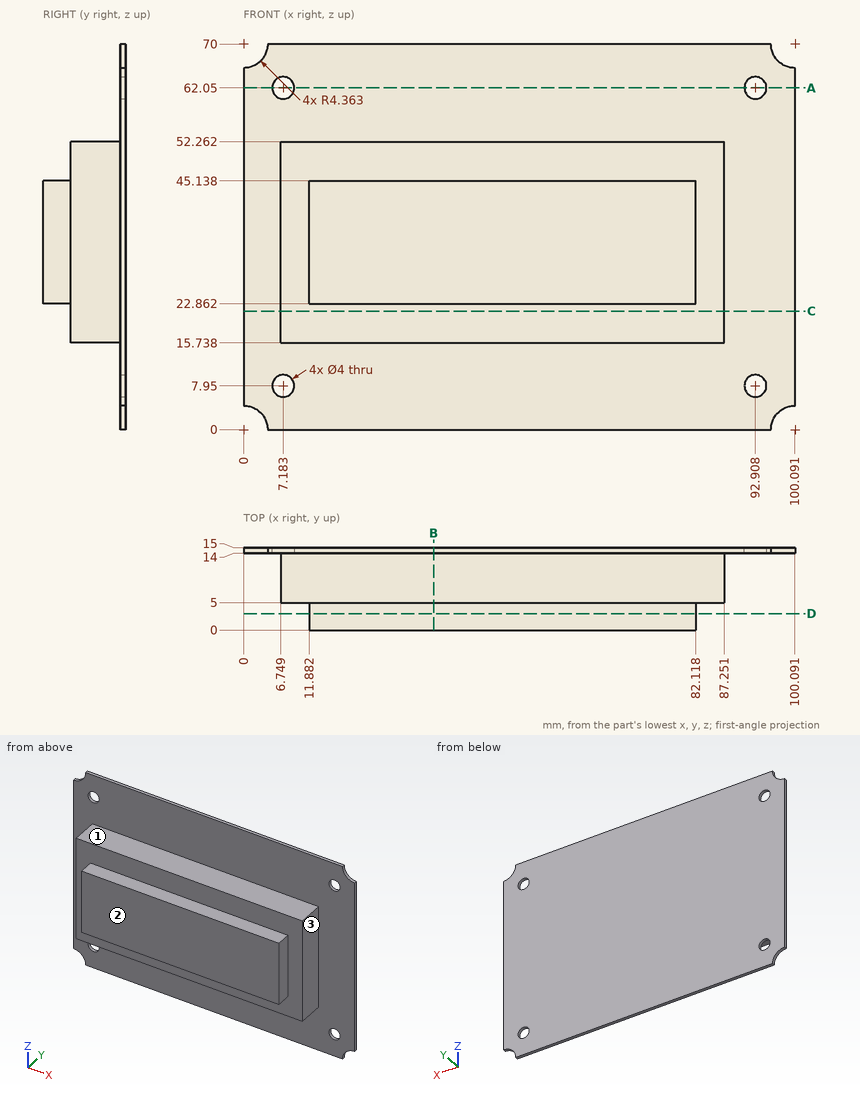
Source: three-view drawing plus pictorial views. Frame: mm from the lowest corner of the part. A direction names the side the tool comes from. Coordinates: 2 decimals unless noted, no trailing zeros. Order: outer loops, then holes, each group sorted by start corner. A loop starts at its lowest first (then second) coordinate and runs counter-clockwise, first axis right, second up.
1) Section A-A (z = 62.05). Return loops of the section in (x, y).
Result sheet:
outline: (0, 14) - (5.18, 14) - (5.18, 15) - (0, 15) - close; (9.18, 14) - (90.91, 14) - (90.91, 15) - (9.18, 15) - close; (94.91, 14) - (100.09, 14) - (100.09, 15) - (94.91, 15) - close
2) Ray query, probe 1 along Z at (x, y) = (84, 12.25); probe 2 along X at (y, z) = (13, 27.5); probe 3 along Y at (x, z) = (75.5, 4.5). Return the intervals inside material, ascending.
Result sheet:
probe 1: z = 15.74 to 52.26
probe 2: x = 6.75 to 87.25
probe 3: y = 14 to 15
3) Section C-C (z = 21.5). Return loops of the section in (x, y).
Result sheet:
outline: (0, 14) - (6.75, 14) - (6.75, 5) - (87.25, 5) - (87.25, 14) - (100.09, 14) - (100.09, 15) - (0, 15) - close
4) Section D-D (y = 3). Return loops of the section in (x, z), then the cut area to 3 significant figures.
Result sheet:
outline: (11.88, 22.86) - (82.12, 22.86) - (82.12, 45.14) - (11.88, 45.14) - close
area: 1,560 mm2
5) Section B-B (x = 34.5). Return loops of the section in (y, z).
Result sheet:
outline: (0, 22.86) - (5, 22.86) - (5, 15.74) - (14, 15.74) - (14, 0) - (15, 0) - (15, 70) - (14, 70) - (14, 52.26) - (5, 52.26) - (5, 45.14) - (0, 45.14) - close
6) First-contact query: P1, Ø4.5, axis at x = 45, y = 9.5, coming from the -Z side; P2, Ø1.5, axis at x = 48.5, y = 2, coming from the +Z side; P3, Ø4, axis at y = 1.5, z = 39.5, coming from the +X side. Flat tips, straight axial feed; report the tip coordinate or a pass-through.
Result sheet:
P1: stops at z = 15.74
P2: stops at z = 45.14
P3: stops at x = 82.12
7) Set-up query: the marked faces 1, 2 and 3. Return all of +Z, -Z, +X, -X, +Y, -Y with unobstructed straight access to the full face (end or side cutting, diameter ignored); none if empty.
Result sheet:
face 1: +Z, +X, -X, -Y
face 2: +Z, -Z, +X, -X, -Y
face 3: +Z, -Z, +X, -Y
